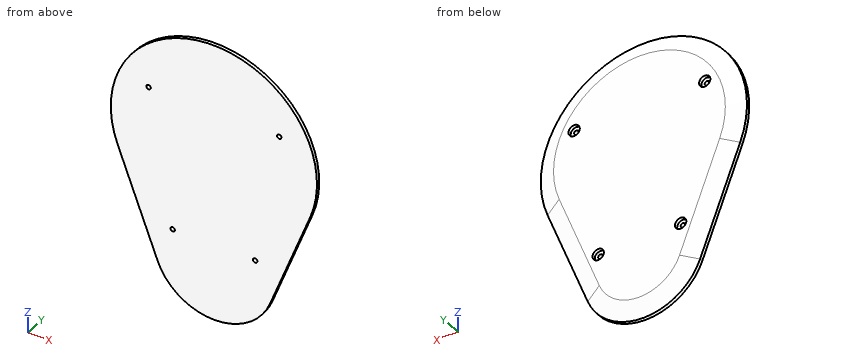
Autodesk Inventor part; units mm, degrees
ref_plane "YZ Plane" through (0, 0, 0) normal (1, 0, 0) x (0, 1, 0)
ref_plane "XZ Plane" through (0, 0, 0) normal (0, 1, 0) x (-1, 0, 0)
ref_plane "XY Plane" through (0, 0, 0) normal (0, 0, 1) x (1, 0, 0)
sketch "Sketch1" plane through (0, 0, 0) normal (0, 1, 0) x (-1, 0, 0)
  arc A0 (28.0215, -10.7143) -> (-28.0215, -10.7143) centre (0, 0) ccw
  arc A1 (14.9976, -25.9821) -> (-16.3459, -41.25) centre (0, -35) ccw construction
  line L0 (0, 0) -> (0, -35) construction
  line L1 (-28.0215, -10.7143) -> (-16.3459, -41.25)
  line L2 (16.3459, -41.25) -> (28.0215, -10.7143)
  arc A2 (14.9976, -25.9821) -> (28.0215, -10.7143) centre (0, 0) ccw construction
  arc A3 (16.3459, -41.25) -> (14.9976, -25.9821) centre (0, -35) ccw construction
  arc A4 (-16.3459, -41.25) -> (16.3459, -41.25) centre (0, -35) ccw
  arc A5 (-28.0215, -10.7143) -> (14.9976, -25.9821) centre (0, 0) ccw construction
  dimension "d0" = 60
  dimension "d1" = 35
  dimension "d2" = 35
extrude "Extrusion1" add sketch "Sketch1" along normal blind 3
chamfer "Chamfer1" distance 5 distance2 2 4 edges at (0, 3, 30) (22.1837, 3, -25.9821) (0, 3, -52.5) (-22.1837, 3, -25.9821) measured on face at (1.8074, 3, 7.3223)
sketch "Sketch2" plane through (0, 3, 0) normal (0, 1, 0) x (1, 0, 0)
  line L0 (-19, -10) -> (19, -10) construction
  line L1 (19, -10) -> (12, 30) construction
  line L2 (12, 30) -> (-12, 30) construction
  line L3 (-12, 30) -> (-19, -10) construction
  circle A0 centre (-19, -10) radius 0.65
  circle A1 centre (19, -10) radius 0.65
  circle A2 centre (-12, 30) radius 0.65
  circle A3 centre (12, 30) radius 0.65
  point P0 (0, 0)
  dimension "d8" = 10
  dimension "d9" = 30
  dimension "d10" = 19
  dimension "d11" = 19
  dimension "d12" = 12
  dimension "d13" = 12
  dimension "d14" = 1.3
  dimension "d15" = 1.3
  dimension "d16" = 1.3
  dimension "d17" = 1.3
extrude "Extrusion2" cut sketch "Sketch2" against normal through all
sketch "Sketch3" plane through (0, 3, 0) normal (0, 1, 0) x (1, 0, 0)
  circle A0 centre (19, -10) radius 0.65
  circle A1 centre (-19, -10) radius 0.65
  arc A2 (-23.3512, 8.9286) -> (23.3512, 8.9286) centre (0, 0) ccw
  line L0 (11.6756, 39.4643) -> (23.3512, 8.9286)
  arc A3 (11.6756, 39.4643) -> (-11.6756, 39.4643) centre (0, 35) ccw
  line L1 (-23.3512, 8.9286) -> (-11.6756, 39.4643)
  circle A4 centre (-19, -10) radius 1.65
  circle A5 centre (19, -10) radius 1.65
  circle A6 centre (12, 30) radius 1.65
  circle A7 centre (-12, 30) radius 1.65
  circle A8 centre (-12, 30) radius 0.65
  circle A9 centre (12, 30) radius 0.65
  dimension "d20" = 3.3
  dimension "d21" = 3.3
  dimension "d22" = 3.3
  dimension "d23" = 3.3
extrude "Extrusion3" cut sketch "Sketch3" against normal blind 1 contours A0 | A1 | A4 | A5 | A6 | A7 | A8 | A9
equation "\"d21\" = d20"
equation "\"d22\" = d20"
equation "\"d23\" = d20"
properties part number "Arm_1_Cover"
CAD build for the part. Positions are in the model's coordinates, mm. Coordinates: 2 decimals unless noted, no trailing zeros. Write each loop counter-clockwise with the first axis right and the second up, starting at its lowest first coordinate (ties: lowest second). Pieces come first, ordered by that corner, then holes. Notation, with made-up numbers: M 47,56 L 91,56 A18 ccw 91,85 Z; hole C 73.25,-3 d7. An arc over 180 degrees is marked long. Answer as a JSON object with one key per item and string values. Group by question number.
1) Saw through at A-A (y = 0.5). Write the cut outline in (x, z).
2) Pin check, flat tips, straight feed: pin 1 Ø1.6 at (x, z) = (11.5, -30.5) entering from +Y; pin 2 Ø0.8 at (x, z) = (-19, 10) entering from +Y. Stop position of each tip, or through.
3) Wall check: line 1 (X direction, y = 0.6, z = 10); line 2 (Z direction, x = 12, y = 0.7); line 3 (Y direction, x = -17, z = -30). Give the ranges that are in metal, low to high. Write a range as from..to.
4) Saw through at C-C (z = -17). Write the cut outline in (x, y), plus the area to 3 significant figures.
5) Saw through at B-B (z = 0). Write the cut outline in (x, y), plus the area to 3 significant figures.
Values follow:
{
 "1": {"outline": "M -28.02,-10.71 L -16.35,-41.25 A17.5 ccw 16.35,-41.25 L 28.02,-10.71 A30 ccw long Z; hole C -19,10 d1.3; hole C -12,-30 d1.3; hole C 12,-30 d1.3; hole C 19,10 d1.3"},
 "2": {"pin 1": "stops at y = 2", "pin 2": "passes through"},
 "3": {"line 1": "x = -28.28..-19.65, -18.35..18.35, 19.65..28.28", "line 2": "z = -47.74..-30.65, -29.35..27.5", "line 3": "y = 0..2.36"},
 "4": {"outline": "M -25.62,0 L 25.62,0 L 25.62,1 L 20.27,3 L -20.27,3 L -25.62,1 Z", "area": "143 mm2"},
 "5": {"outline": "M -30,0 L 30,0 L 30,1 L 25,3 L -25,3 L -30,1 Z", "area": "170 mm2"}
}
